from build123d import *

# Parameters (mm, degrees)
F0_R     = 11
F1_DEPTH = 3


with BuildPart() as f1:
    # F0 (on Front) → F1 (new body, symmetric)
    with BuildSketch(Plane.XZ):
        with BuildLine():
            ThreePointArc((13.091594, 35.215377), (15.413694, 40.839465), (10.585045, 44.541717))
            Line((10.585045, 44.541717), (-5.556075, 44.541717))
            ThreePointArc((-5.556075, 44.541717), (-9.068174, 43.100531), (-10.555639, 39.607781))
            ThreePointArc((-10.555639, 39.607781), (-11.098737, 32.23023), (-12.52502, 24.971516))
            ThreePointArc((-12.52502, 24.971516), (-24.124845, 5.691327), (-39.579164, -10.662439))
            ThreePointArc((-39.579164, -10.662439), (-41.860242, -13.696996), (-41.352296, -17.459156))
            Line((-41.352296, -17.459156), (-33.281736, -31.437776))
            ThreePointArc((-33.281736, -31.437776), (-27.661168, -33.768383), (-23.951614, -28.945342))
            ThreePointArc((-23.951614, -28.945342), (-23.944714, -28.112998), (-23.926531, -27.280824))
            ThreePointArc((-23.926531, -27.280824), (-4.469508, -23.436159), (15.363457, -23.332743))
            ThreePointArc((15.363457, -23.332743), (22.362829, -25.726903), (29.023525, -28.945342))
            ThreePointArc((29.023525, -28.945342), (32.792068, -29.403535), (35.79622, -27.082561))
            Line((35.79622, -27.082561), (43.86678, -13.10394))
            ThreePointArc((43.86678, -13.10394), (43.074861, -7.071082), (37.043208, -6.270036))
            ThreePointArc((37.043208, -6.270036), (35.274041, -7.249485), (33.473584, -8.170152))
            ThreePointArc((33.473584, -8.170152), (19.248618, 11.113195), (9.661233, 33.07405))
            ThreePointArc((9.661233, 33.07405), (11.358782, 34.172958), (13.091594, 35.215377))
        make_face()
        Polygon((-30.615118, -21.017243), (-34.27078, -15.948025), (-31.748977, -10.276928), (-25.576762, -9.625325), (-22.943373, -13.246362), (-21.926349, -14.64482), (-24.442903, -20.36564), align=None, mode=Mode.SUBTRACT)
        Circle(F0_R, mode=Mode.SUBTRACT)
        Polygon((22.943373, -13.246362), (25.576762, -9.625325), (31.748977, -10.276928), (34.265531, -15.997749), (30.615118, -21.017243), (24.442903, -20.36564), (21.926349, -14.64482), align=None, mode=Mode.SUBTRACT)
        Polygon((6.182559, 32.802254), (3.792685, 27.043044), (0.003247, 26.546629), (-2.389875, 26.233131), (-6.182559, 31.182428), (-3.792685, 36.941638), (2.389875, 37.751551), align=None, mode=Mode.SUBTRACT)
    extrude(amount=F1_DEPTH, both=True)


solid = f1.part
Design review of the part built by this model. Coordinates are the model's own, in mm. A direction names the side the tool comes from. Give positions to 0.01 mm unless a question says otherwise; leave off trailing zeros. Order: outer loops, then holes, each group sorted by start corner. A loop starts at its lowest first (then second) coordinate and runs counter-clockwise, first axis right, second up. Notation, with made-up numbers: (75, -34.5) - (107, -34.5) arc R16 ccw to (107, -27.5) - close; hole circle Ø6 at (-18.5, -18). An arc over 180 degrees is marked (long way). Write item = value, one per line. Start each with the question number.
Q1. We need section C-C on x = 20.5. State the section outline as (y, z) points, plus the area to 3 significant figures.
Q2. Mouldability with a two-part tool opening along Z and no side actions: class faces 4 (the face through (-41.846, -0.042, -13.644)), 5 (the face through (35.299, -0.042, -7.236)), 6 (the face through (19.42, -0.04, 10.82)) as released by +Z, released by -Z, zero draft, split by the parting line, or undercut.
Q3. Tool access review of faces 1 (the face through (22.3, 0, -25.7)), 2 (the face through (4.26, -0.04, 35.31)), 3 (the face through (1, -3, -12)): name each direction out of +Z, -Z, +X, -X, +Y, -Y from which nothing blocks a thin tool from reaching the whole face with its end or side.
Q4. To check wall thickness, follow L1, parallel to X at y = 1.75, z = -17; L2, parallel to Z at x = 0, y = -0.85; L3, parallel to X at y = 0.25, z = -14.5. State the ranges of each line that lie inside material, in increasing order. Write a range as from..to.
Q5. We need section B-B on y = -1.75. State how many separate pieces and enclosed holes the cut face has, plus the area to 3 significant figures.
Q6. We need section D-D on z = 21.5. State the section outline as (x, y) points, plus the area to 3 significant figures.
Q7. We need section A-A on z = 0. State the section outline as (x, y) points, plus the area to 3 significant figures.
Q8. Clearance check with flat-ended pins moving along their axes: pin 1 Ø1 at (x, y) = (-21, 0) entering from -Z; pin 2 Ø1 at (x, y) = (-30.5, 0.5) entering from +Z; pin 3 Ø1 at (y, z) = (-0.5, 35) entering from +X. State where each tip first meets the part, or that it passes through.
Working result:
q1.outline = (-3, -25) - (3, -25) - (3, 9) - (-3, 9) - close
q1.area = 204 mm²
q2.face_4 = split by the parting line
q2.face_5 = released by +Z
q2.face_6 = undercut
q3.face_1 = -Z, +Y, -Y
q3.face_2 = +Y, -Y
q3.face_3 = +Z, -Z, +X, -X, -Y
q4.L1 = -41.59..-33.51, -22.96..22.96, 33.54..41.62
q4.L2 = -23.08..-11, 11..26.55, 37.44..44.54
q4.L3 = -42..-33.63, -22.03..22.03, 33.61..43.06
q5.separate_pieces = 1
q5.enclosed_holes = 4
q5.area = 2,730 mm²
q6.outline = (-14.21, -3) - (13.98, -3) - (13.98, 3) - (-14.21, 3) - close
q6.area = 169 mm²
q7.outline = (-28.77, -3) - (-11, -3) - (-11, 3) - (-28.77, 3) - close; (11, -3) - (26.62, -3) - (26.62, 3) - (11, 3) - close
q7.area = 200 mm²
q8.pin_1 = -26.59
q8.pin_2 = -1.38
q8.pin_3 = 13.53
